Could you check a few things on this drawing? It's one solid part, dimensions in mm from its lowest x, y, z. A direction names the side the tool comes from. Give positions to 0.01 mm unless a question says otherwise; leave off trailing zeros. Write each loop counter-clockwise with the first axis right and the second up, starting at its lowest first coordinate (ties: lowest second). Pieces come first, ordered by that corner, then holes. Notation, with made-up numbers: M -2,69.25 L 24,69.25 A11 ccw 24,78.25 Z; hole C 16.25,64.5 d3. An arc over 180 degrees is marked long. Write each question's results on one line, items separated by ' | '.
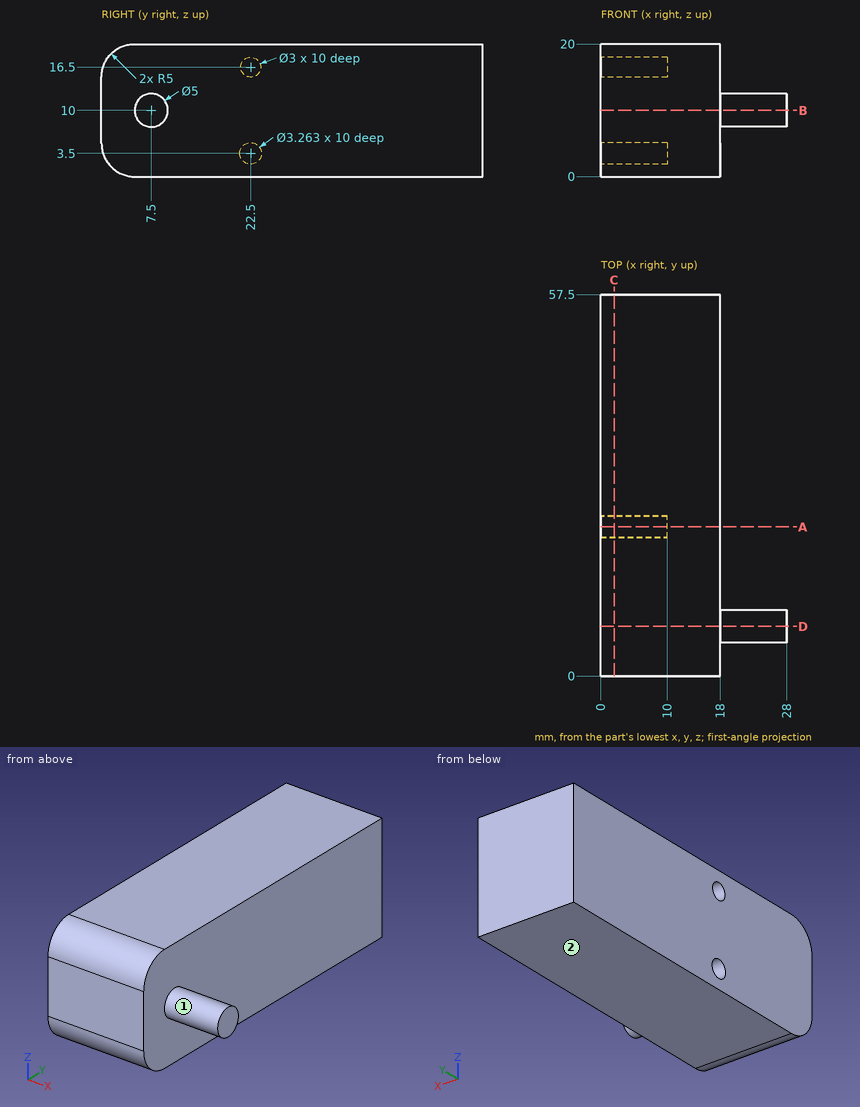
Item 1: If I drill on line 1 (Z direction, x = 6.5, y = 22.5); line 2 (X direction, y = 27.5, z = 13.5); line 3 (Y direction, x = 14.25, z = 18.5), over which ranges is the centre line in solid material (lowest first)? Write a range as from..to.
Geometry says:
line 1: z = 0..1.87, 5.13..15, 18..20 | line 2: x = 0..18 | line 3: y = 1.43..57.5
Item 2: I'm going to push flat-ended pins straight in: pin 1 (1.5 mm diameter, centred on x = 6.5, z = 10, fed in from -Y); pin 2 (3 mm diameter, centred on y = 17, z = 14.5, fed in from +X); pin 3 (3 mm diameter, centred on x = 20, z = 12.5, fed in from +Y); pin 4 (1.5 mm diameter, centred on y = 23, z = 16, fed in from -X). Where does each tip first touch, or does it pass through?
Geometry says:
pin 1: stops at y = 0 | pin 2: stops at x = 18 | pin 3: stops at y = 9.79 | pin 4: stops at x = 10
Item 3: I want a section at A-A, the plane y = 22.5. Please give me the cut outline in (x, z), and give its area (3 significant figures).
Geometry says:
outline: M 0,0 L 18,0 L 18,20 L 0,20 L 0,18 L 10,18 L 10,15 L 0,15 L 0,5.13 L 10,5.13 L 10,1.87 L 0,1.87 Z | area: 297 mm2
Item 4: For the marked faces 1 and 2, which set-ups out of +Z, -Z, +X, -X, +Y, -Y let a thin tool reach every point of the face, with its end or its side?
Geometry says:
face 1: +X | face 2: -Z, +X, -X, +Y, -Y
Item 5: I want a section at B-B, the plane z = 10. Please give me the cut outline in (x, y).
Geometry says:
outline: M 0,0 L 18,0 L 18,5 L 28,5 L 28,10 L 18,10 L 18,57.5 L 0,57.5 Z
Item 6: I want a section at C-C, the plane x = 2. Please give me the cut outline in (y, z), and give its area (3 significant figures).
Geometry says:
outline: M 0,5 A5 ccw 5,0 L 57.5,0 L 57.5,20 L 5,20 A5 ccw 0,15 Z; hole C 22.5,3.5 d3.26; hole C 22.5,16.5 d3 | area: 1,120 mm2
Item 7: I want a section at D-D, the plane y = 7.5. Please give me the cut outline in (x, z).
Geometry says:
outline: M 0,0 L 18,0 L 18,7.5 L 28,7.5 L 28,12.5 L 18,12.5 L 18,20 L 0,20 Z
